```python
from build123d import *

# Parameters (mm, degrees)
PAD_DEPTH    = 20
THICKNESS_T  = -4
FILLET_R     = 4
FILLET001_R  = 2
CHAMFER_SIZE = 0.5


with BuildPart() as part:
    # Sketch → Pad (new body)
    with BuildSketch(Plane.XY):
        Polygon((-47.5, 20), (-27.5, 20), (-27.5, 7.5), (27.5, 7.5), (27.5, 20), (47.5, 20), (47.5, -20), (27.5, -20), (27.5, -7.5), (-27.5, -7.5), (-27.5, -20), (-47.5, -20), align=None)
    extrude(amount=PAD_DEPTH)

    # Thickness
    thickness_openings = [part.faces().sort_by_distance(p)[0] for p in [
        (0, 0, 0),
        (0, 0, 20),
    ]]
    offset(amount=THICKNESS_T, openings=thickness_openings)

    # Fillet
    fillet_edges = [part.edges().sort_by_distance(p)[0] for p in [
        (-47.5, -20, 10),
        (-27.5, -20, 10),
        (27.5, -20, 10),
        (47.5, -20, 10),
        (47.5, 20, 10),
        (27.5, 20, 10),
        (-27.5, 20, 10),
        (-47.5, 20, 10),
    ]]
    fillet(fillet_edges, radius=FILLET_R)

    # Fillet001
    fillet001_edges = [part.edges().sort_by_distance(p)[0] for p in [
        (-27.5, -7.5, 10),
        (-27.5, 7.5, 10),
        (27.5, 7.5, 10),
        (27.5, -7.5, 10),
        (-43.5, 16, 10),
        (-31.5, 16, 10),
        (-31.5, -16, 10),
        (-43.5, -16, 10),
        (31.5, 16, 10),
        (43.5, 16, 10),
        (31.5, -16, 10),
        (43.5, -16, 10),
    ]]
    fillet(fillet001_edges, radius=FILLET001_R)

    # Chamfer
    chamfer_edges = [part.edges().sort_by_distance(p)[0] for p in [
        (-27.5, 12.75, 20),
        (-26.914214, 8.085786, 20),
        (-28.671573, 18.828427, 20),
        (0, 7.5, 20),
        (-37.5, 20, 20),
        (26.914214, 8.085786, 20),
        (-46.328427, 18.828427, 20),
        (27.5, 12.75, 20),
        (-47.5, 0, 20),
        (28.671573, 18.828427, 20),
        (-46.328427, -18.828427, 20),
        (37.5, 20, 20),
        (-37.5, -20, 20),
        (46.328427, 18.828427, 20),
        (-28.671573, -18.828427, 20),
        (47.5, 0, 20),
        (-27.5, -12.75, 20),
        (46.328427, -18.828427, 20),
        (-26.914214, -8.085786, 20),
        (37.5, -20, 20),
        (0, -7.5, 20),
        (28.671573, -18.828427, 20),
        (26.914214, -8.085786, 20),
        (27.5, -12.75, 20),
        (-37.5, -16, 20),
        (-32.085786, -15.414214, 20),
        (-42.914214, -15.414214, 20),
        (-31.5, -10.75, 20),
        (-43.5, 0, 20),
        (-30.328427, -4.671573, 20),
        (-42.914214, 15.414214, 20),
        (0, -3.5, 20),
        (-37.5, 16, 20),
        (30.328427, -4.671573, 20),
        (-32.085786, 15.414214, 20),
        (31.5, -10.75, 20),
        (-31.5, 10.75, 20),
        (32.085786, -15.414214, 20),
        (-30.328427, 4.671573, 20),
        (37.5, -16, 20),
        (0, 3.5, 20),
        (42.914214, -15.414214, 20),
        (30.328427, 4.671573, 20),
        (43.5, 0, 20),
        (31.5, 10.75, 20),
        (42.914214, 15.414214, 20),
        (32.085786, 15.414214, 20),
        (37.5, 16, 20),
        (-27.5, 12.75, 0),
        (-26.914214, 8.085786, 0),
        (-28.671573, 18.828427, 0),
        (0, 7.5, 0),
        (-37.5, 20, 0),
        (26.914214, 8.085786, 0),
        (-46.328427, 18.828427, 0),
        (27.5, 12.75, 0),
        (-47.5, 0, 0),
        (28.671573, 18.828427, 0),
        (-46.328427, -18.828427, 0),
        (37.5, 20, 0),
        (-37.5, -20, 0),
        (46.328427, 18.828427, 0),
        (-28.671573, -18.828427, 0),
        (47.5, 0, 0),
        (-27.5, -12.75, 0),
        (46.328427, -18.828427, 0),
        (-26.914214, -8.085786, 0),
        (37.5, -20, 0),
        (0, -7.5, 0),
        (28.671573, -18.828427, 0),
        (26.914214, -8.085786, 0),
        (27.5, -12.75, 0),
        (-37.5, -16, 0),
        (-32.085786, -15.414214, 0),
        (-42.914214, -15.414214, 0),
        (-31.5, -10.75, 0),
        (-43.5, 0, 0),
        (-30.328427, -4.671573, 0),
        (-42.914214, 15.414214, 0),
        (0, -3.5, 0),
        (-37.5, 16, 0),
        (30.328427, -4.671573, 0),
        (-32.085786, 15.414214, 0),
        (31.5, -10.75, 0),
        (-31.5, 10.75, 0),
        (32.085786, -15.414214, 0),
        (-30.328427, 4.671573, 0),
        (37.5, -16, 0),
        (0, 3.5, 0),
        (42.914214, -15.414214, 0),
        (30.328427, 4.671573, 0),
        (43.5, 0, 0),
        (31.5, 10.75, 0),
        (42.914214, 15.414214, 0),
        (32.085786, 15.414214, 0),
        (37.5, 16, 0),
    ]]
    chamfer(chamfer_edges, length=CHAMFER_SIZE)


solid = part.part
```
The listing builds one solid part. Answer for the finished solid, in the listing's coordinates (mm). A direction names the side the tool comes from. Round coordinates to 2 decimals unless told otherwise and drop trailing zeros. Order: outer loops, then holes, each group sorted by start corner. A loop starts at its lowest first (then second) coordinate and runs counter-clockwise, first axis right, second up. Notation, with made-up numbers: (7, 85.25) -> (52, 85.25) arc R29 cw to (52, 119.25) -> close; hole circle Ø2 at (89.25, -21.5). An arc over 180 degrees is marked (long way). Answer as CSV lines item,"result". Start each with the question number.
(1) For a pull along Y with two mould halves and no side action, classify faces 1 (the face through (28.95, -18.6, 0.14)), 2 (the face through (46.297, 18.859, 10.133)), 3 (the face through (32.007, -15.526, 0.365)), 4 (the face through (-32, 15.53, 19.64)) as +Y half, -Y half, draft (parallel to the pull), parting line (faces both ways), or undercut.
(2) A tool of negligible diameter and unlimited length cuts with its end or side. For faces 5 (the face through (-28.958, 18.599, 19.865)), 6 (the face through (-43.026, 15.493, 0.365)), 7 (the face through (-43, -15.53, 19.64)), 8 (the face through (-32.07, 15.4, 9.87)), from which of +Z, -Z, +X, -X, +Y, -Y can it reach the whole face along a straight path? Write none if from no direction.
(3) Find the intervals of material crossed by probe 1 along X at (y, z) = (-11.5, 12); probe 2 along Y at (x, z) = (-10, 14); probe 3 along X at (y, z) = (3, 6.5), in increasing order. Write a range as from..to.
(4) The part is cut by section C-C (y = -8.5). Count the separate pieces of the cut face and the enclosed holes in it, then the cut area to 3 significant figures.
(5) Flat-ended cylindrical pins translate along their axes: pin 1 Ø2 at (x, z) = (-9, 13.5) entering from +Y; pin 2 Ø12 at (x, z) = (20.5, 9) entering from -Y; pin 3 Ø12 at (x, z) = (14.5, 13) entering from -Y. Find the tip coordinate at first contact, or state that the pin passes through.
(6) The part is cut by section A-A (y = 1). Determine the outline of the cut face in (x, z).
(7) The part is cut by section B-B (x = -22.5). Determine the outline of the cut face in (y, z).
Evaluation:
1,face 1,"-Y half"
1,face 2,"+Y half"
1,face 3,"undercut"
1,face 4,"undercut"
2,face 5,"+Z, +Y"
2,face 6,"-Z"
2,face 7,"+Z"
2,face 8,"+Z, -Z"
3,probe 1,"-47.5..-43.5, -31.5..-27.5, 27.5..31.5, 43.5..47.5"
3,probe 2,"-7.5..-3.5, 3.5..7.5"
3,probe 3,"-47.5..-43.5, 43.5..47.5"
4,separate pieces,"4"
4,enclosed holes,"0"
4,area,"329 mm²"
5,pin 1,"y = 7.5"
5,pin 2,"y = -7.77"
5,pin 3,"y = -7.5"
6,outline,"(-47.5, 0.5) -> (-47, 0) -> (-44, 0) -> (-43.5, 0.5) -> (-43.5, 19.5) -> (-44, 20) -> (-47, 20) -> (-47.5, 19.5) -> close; (43.5, 0.5) -> (44, 0) -> (47, 0) -> (47.5, 0.5) -> (47.5, 19.5) -> (47, 20) -> (44, 20) -> (43.5, 19.5) -> close"
7,outline,"(-7.5, 0.5) -> (-7, 0) -> (-4, 0) -> (-3.5, 0.5) -> (-3.5, 19.5) -> (-4, 20) -> (-7, 20) -> (-7.5, 19.5) -> close; (3.5, 0.5) -> (4, 0) -> (7, 0) -> (7.5, 0.5) -> (7.5, 19.5) -> (7, 20) -> (4, 20) -> (3.5, 19.5) -> close"
